Geometry check sheet. Reference: the model listing, model coordinates, mm. Face numbers are marked on the shaded views. A direction names the side the tool comes from. Round coordinates to 2 decimals unless told otherwise and drop trailing zeros. Order: outer loops, then holes, each group sorted by start corner. A loop starts at its lowest first (then second) coordinate and runs counter-clockwise, first axis right, second up. Notation, with made-up numbers: (48.5, 61.25) -> (99.5, 61.25) arc R23 cw to (99.5, 92.25) -> close; hole circle Ø6 at (-35, 13). An arc over 180 degrees is marked (long way). Use a Markdown table: item, result. Add a question column.
Item 1: Sectioned sample at D-D, the plane z = 4.5. Record the cut outline in (x, y).
Item 2: Set-up check for the marked faces 1 and 2: record each of +Z, -Z, +X, -X, +Y, -Y from which the full face is reachable in a straight line by a thin tool's end or side.
Item 3: Mould release check, pull along X, two halves, no side actions. Record for the marked faces 3, 4, 5 and 6: pulls with the +X half, pulls with the -X half, needs draft (parallel to the pull), parting line crosses it, or undercut.
Item 4: Sectioned sample at C-C, the plane y = -2.05. Record the cut outline in (x, z).
Item 5: Gauge pin test, flat ends, axial feed: pin 1 Ø0.6 at (x, z) = (4.5, -10.5) entering from -Y; pin 2 Ø0.5 at (x, z) = (0.5, -11) entering from +Y; pin 3 Ø1 at (x, z) = (-1, -8.5) entering from +Y. Record the tip position at first contact, or that the pin passes through.
Item 6: Sectioned sample at B-B, the plane x = -4.5. Record the cut outline in (y, z).
Item 7: Sectioned sample at A-A, the plane z = 10. Record the cut outline in (x, y).
Item 8: Material ranges on probe 1 along Z at (x, y) = (-5.25, -3.4); probe 2 along Z at (x, y) = (-4.5, -5.35); probe 3 along X at (y, z) = (-4.7, -10), recorded low to high. Write a range as [from, to].
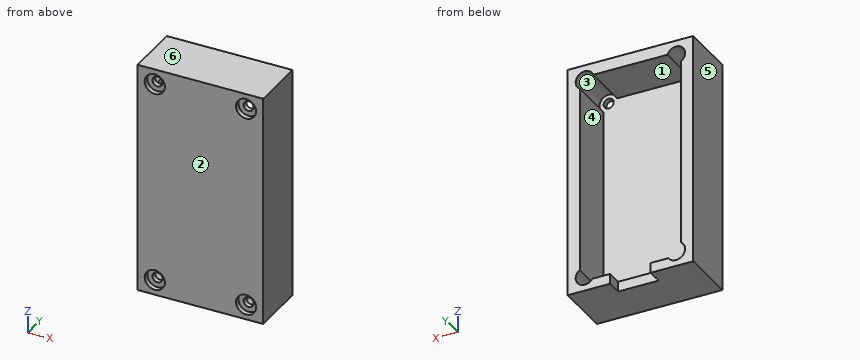
Autodesk Inventor part; units mm, degrees
ref_plane "YZ Plane" through (0, 0, 0) normal (1, 0, 0) x (0, 1, 0)
ref_plane "XZ Plane" through (0, 0, 0) normal (0, 1, 0) x (-1, 0, 0)
ref_plane "XY Plane" through (0, 0, 0) normal (0, 0, 1) x (1, 0, 0)
sketch "Эскиз1" plane through (0, 0, 0) normal (0, 1, 0) x (-1, 0, 0)
  line L0 (6.2, 11.5) -> (-6.2, 11.5)
  line L1 (-6.2, 11.5) -> (-6.2, -11.5)
  line L2 (-6.2, -11.5) -> (6.2, -11.5)
  line L3 (6.2, -11.5) -> (6.2, 11.5)
  line L4 (6.2, 11.5) -> (-6.2, -11.5) construction
  line L5 (-6.2, 11.5) -> (6.2, -11.5) construction
  point P0 (0, 0)
  dimension "d0" = 12.4
  dimension "d1" = 23
extrude "Выдавливание1" add sketch "Эскиз1" against normal blind 5.5
sketch "Эскиз2" plane through (0, 0, 0) normal (0, 1, 0) x (1, 0, 0)
  line L0 (-6.2, -11.5) -> (6.2, -11.5)
  line L1 (6.2, -11.5) -> (6.2, 11.5)
  line L2 (6.2, 11.5) -> (-6.2, 11.5)
  line L3 (-6.2, 11.5) -> (-6.2, -11.5)
  line L4 (-5, 10.5) -> (5, 10.5)
  line L5 (5, 10.5) -> (5, -10.3)
  line L6 (5, -10.3) -> (-5, -10.3)
  line L7 (-5, -10.3) -> (-5, 10.5)
  line L8 (0, 16.1) -> (0, -16.1)
  line L9 (-8.68, 0) -> (8.68, 0)
  point P0 (0, 0)
  dimension "d4" = 1
  dimension "d5" = 1.2
extrude "Выдавливание2" cut sketch "Эскиз2" against normal blind 4.5 contours L8 L9 L5 L6 | L6 L7 L9 L8 | L7 L4 L8 L9 | L8 L4 L5 L9
sketch "Эскиз3" plane through (0, 0, 0) normal (0, 1, 0) x (1, 0, 0)
  line L0 (-4.5, -10) -> (4.5, -10)
  line L1 (4.5, -10) -> (4.5, 10)
  line L2 (4.5, 10) -> (-4.5, 10)
  line L3 (-4.5, 10) -> (-4.5, -10)
  line L4 (-4.5, -10) -> (4.5, 10) construction
  line L5 (4.5, -10) -> (-4.5, 10) construction
  point P0 (0, 0)
  dimension "d8" = 9
  dimension "d9" = 20
hole "Отверстие1" at (-4.5, 0, -10) at (4.5, 0, -10) at (4.5, 0, 10) at (-4.5, 0, 10) direction (0, -1, 0) diameter 1 depth 8 tip angle 118 counterbore diameter 1.8 counterbore depth 4.5
sketch "Эскиз4" plane through (0, -5.5, 0) normal (0, -1, 0) x (1, 0, 0)
  circle A0 centre (-4.5, 10) radius 0.5
  circle A1 centre (4.5, 10) radius 0.5
  circle A2 centre (4.5, -10) radius 0.5
  circle A3 centre (-4.5, -10) radius 0.5
  circle A4 centre (-4.5, 10) radius 1
  circle A5 centre (4.5, 10) radius 1
  circle A6 centre (4.5, -10) radius 1
  circle A7 centre (-4.5, -10) radius 1
  point P0 (0, 0)
  dimension "d17" = 2
extrude "Выдавливание3" cut sketch "Эскиз4" against normal blind 0.5
sketch "Эскиз5" plane through (0, 0, 0) normal (0, 1, 0) x (1, 0, 0)
  line L0 (-2, 10.5) -> (2, 10.5)
  line L1 (2, 10.5) -> (2, 11.5)
  line L2 (2, 11.5) -> (-2, 11.5)
  line L3 (-2, 11.5) -> (-2, 10.5)
  arc A0 (3.6515, -10.3) -> (5, -9.2517) centre (4.5, -10) ccw
  line L4 (3.6515, -10.3) -> (-3.6515, -10.3)
  arc A1 (-5, -9.2517) -> (-3.6515, -10.3) centre (-4.5, -10) ccw
  line L5 (-5, -9.2517) -> (-5, 9.2517)
  arc A2 (-3.7517, 10.5) -> (-5, 9.2517) centre (-4.5, 10) ccw
  line L6 (-3.7517, 10.5) -> (3.7517, 10.5)
  arc A3 (5, 9.2517) -> (3.7517, 10.5) centre (4.5, 10) ccw
  line L7 (5, 9.2517) -> (5, -9.2517)
  line L8 (-6.2, -11.5) -> (6.2, -11.5)
  line L9 (6.2, -11.5) -> (6.2, 11.5)
  line L10 (6.2, 11.5) -> (-6.2, 11.5)
  line L11 (-6.2, 11.5) -> (-6.2, -11.5)
  line L12 (0, 16.1) -> (0, -16.1)
  point P0 (0, 0)
  point P1 (0, 11.5)
  point P2 (0, 10.5)
  dimension "d23" = 4
extrude "Выдавливание4" cut sketch "Эскиз5" against normal blind 1.5 contours L3 L2 L12 L0 | L12 L2 L1 L0
properties part number "Крышка корпуса задняя" material "Пластик ПК/АБС"
Found:
| question | item | result |
|---|---|---|
| 1 | outline | (-6.2, -5.5) -> (6.2, -5.5) -> (6.2, 0) -> (5, 0) -> (5, -4.5) -> (-5, -4.5) -> (-5, 0) -> (-6.2, 0) -> close |
| 2 | face 1 | +Y |
| 2 | face 2 | +Z, -Z, +X, -X, -Y |
| 3 | face 3 | undercut |
| 3 | face 4 | undercut |
| 3 | face 5 | pulls with the -X half |
| 3 | face 6 | needs draft |
| 4 | outline | (-6.2, -11.5) -> (6.2, -11.5) -> (6.2, 11.5) -> (-6.2, 11.5) -> close; hole (-5, -9.25) arc R0.9 ccw (long way) to (-3.75, -10.5) -> (3.75, -10.5) arc R0.9 ccw (long way) to (5, -9.25) -> (5, 9.25) arc R0.9 ccw (long way) to (3.65, 10.3) -> (-3.65, 10.3) arc R0.9 ccw (long way) to (-5, 9.25) -> close |
| 5 | pin 1 | stops at y = -5 |
| 5 | pin 2 | stops at y = -1.5 |
| 5 | pin 3 | stops at y = -4.5 |
| 6 | outline | (-5.5, -11.5) -> (0, -11.5) -> (0, -10.9) -> (-4.5, -10.9) -> (-4.5, -10.5) -> (-5, -10.5) -> (-5, -11) -> (-5.5, -11) -> close; (-5.5, -9) -> (-5, -9) -> (-5, -9.5) -> (-4.5, -9.5) -> (-4.5, 9.5) -> (-5, 9.5) -> (-5, 9) -> (-5.5, 9) -> close; (-5.5, 11) -> (-5, 11) -> (-5, 10.5) -> (-4.5, 10.5) -> (-4.5, 10.9) -> (0, 10.9) -> (0, 11.5) -> (-5.5, 11.5) -> close |
| 7 | outline | (-6.2, -5.5) -> (-5.5, -5.5) -> (-5.5, -5) -> (-5, -5) -> (-5, -4.5) -> (-5.4, -4.5) -> (-5.4, 0) -> (-6.2, 0) -> close; (-4, -5) -> (-3.5, -5) -> (-3.5, -5.5) -> (3.5, -5.5) -> (3.5, -5) -> (4, -5) -> (4, -4.5) -> (-4, -4.5) -> close; (5, -5) -> (5.5, -5) -> (5.5, -5.5) -> (6.2, -5.5) -> (6.2, 0) -> (5.4, 0) -> (5.4, -4.5) -> (5, -4.5) -> close |
| 8 | probe 1 | z = [-11.5, -10.5], [-9.5, 9.5], [10.5, 11.5] |
| 8 | probe 2 | z = [-11.5, -11], [-9, 9], [11, 11.5] |
| 8 | probe 3 | x = [-6.2, -5], [-4, 4], [5, 6.2] |
